from build123d import *

# Parameters (mm, degrees)
SKETCH_W       = 12
SKETCH_H       = 17.5
PAD_DEPTH      = 1.5
PAD_DEPTH_BACK = 10
SKETCH001_R    = 0.75
PAD001_DEPTH   = 10
PAD002_DEPTH   = 5
FILLET_R       = 1
FILLET001_R    = 1
FILLET002_R    = 1
SKETCH003_W    = 5.5
SKETCH003_H    = 7
PAD003_DEPTH   = 1.8
SKETCH004_R    = 2
PAD004_DEPTH   = 0.5
SKETCH005_R    = 2
PAD005_DEPTH   = 7
PAD005_TAPER   = -60


with BuildPart() as part:
    # Sketch → Pad (new body, two sides)
    with BuildSketch(Plane.XY) as pad_sk:
        Rectangle(SKETCH_W, SKETCH_H)
    extrude(amount=PAD_DEPTH)
    extrude(pad_sk.sketch, amount=-PAD_DEPTH_BACK)

    # Sketch001 → Pad001 (join)
    with BuildSketch(Plane.XY):
        with Locations((-3.25, 6)):
            Circle(SKETCH001_R)
        with Locations((-3.25, -6)):
            Circle(SKETCH001_R)
    extrude(amount=PAD001_DEPTH)

    # Sketch002 → Pad002 (join, symmetric)
    with BuildSketch(Plane.XZ):
        with BuildLine():
            ThreePointArc((16, -10), (13.071068, -2.928932), (6, 0))
            Line((6, -10), (6, 0))
            Line((16, -10), (6, -10))
        make_face()
    extrude(amount=PAD002_DEPTH, both=True)

    # Fillet
    fillet_edges = [part.edges().sort_by_distance(p)[0] for p in [
        (6, -8.75, -4.25),
        (-6, -8.75, -4.25),
        (6, 8.75, -4.25),
        (-6, 8.75, -4.25),
    ]]
    fillet(fillet_edges, radius=FILLET_R)

    # Fillet001
    fillet001_edges = [part.edges().sort_by_distance(p)[0] for p in [
        (13.071068, -5, -2.928932),
        (13.071068, 5, -2.928932),
    ]]
    fillet(fillet001_edges, radius=FILLET001_R)

    # Fillet002
    fillet002_edges = [part.edges().sort_by_distance(p)[0] for p in [
        (6, -5, -5.5),
    ]]
    fillet(fillet002_edges, radius=FILLET002_R)

    # Sketch003 (on Face6 of Fillet002) → Pad003 (join)
    with BuildSketch(Plane.XY.offset(1.5)):
        with Locations((-3.25, 0)):
            Rectangle(SKETCH003_W, SKETCH003_H)
    extrude(amount=PAD003_DEPTH)

    # Sketch004 (on Face28 of Pad003) → Pad004 (join)
    with BuildSketch(Plane.XY.offset(3.3)):
        with Locations((-3.25, -0.25)):
            Circle(SKETCH004_R)
    extrude(amount=PAD004_DEPTH)

    # Sketch005 (on Face32 of Pad004) → Pad005 (join)
    with BuildSketch(Plane.XY.offset(3.8)):
        with Locations((-3.25, -0.25)):
            Circle(SKETCH005_R)
    extrude(amount=PAD005_DEPTH, taper=PAD005_TAPER)

    # Sketch006 (on DatumPlane) → Groove (revolve, cut)
    with BuildSketch(Plane(origin=(-3.25, -0.25, 3.8), x_dir=(1, 0, 0), z_dir=(0, -1, 0))):
        Polygon((2, 0), (2, -18), (30, -18), (30, 7), (14.124356, 7), align=None)
    revolve(axis=Axis((-3.25, -0.25, 3.8), (0, 0, 1)), mode=Mode.SUBTRACT)


solid = part.part
Can you work these out from the model? Positions are in its coordinate system, mm. A direction names the side the tool comes from. Coordinates: 2 decimals unless noted, no trailing zeros. Write each loop counter-clockwise with the first axis right and the second up, starting at its lowest first coordinate (ties: lowest second). Pieces come first, ordered by that corner, then holes.
Q1. For P1, Ø1, axis at x = -4.5, y = -7.5, coming from the -Z side; P2, Ø4, axis at y = -0.5, z = 6, coming from the -X side; P3, Ø3, axis at x = -14, z = 7, coming from the +Y side; P4, Ø4, axis at x = 5.5, y = 0, coming from the -Z side, each with a flat end and sliding along its axis, tell me the tip position at first contact or that it passes through.
Results found:
P1: stops at z = 6.6
P2: stops at x = -12.52
P3: passes through
P4: stops at z = 6.54
Q2. Which directions (+Z, -Z, +X, -X, +Y, -Y) give clear straight access to the entire face, cutting with the end or side of a thin tool? Please do faces 1 (the face through (-3, 0, 10.8)), 2 (the face through (-3.7, -2.2, -3.2)).
Results found:
face 1: +Z, +X, -X, +Y, -Y
face 2: -Z
Q3. Please list where these lines run through material, in increasing order: L1, parallel to Z at x = 0.5, y = -6.5; L2, parallel to Z at x = 8.5, y = -4.25; L3, parallel to X at y = -1, z = 0.
Results found:
L1: z = 6.85 to 10.8
L2: z = 9.81 to 10.8
L3: x = -5.1 to -1.4
Q4. Imagine slicing it at A-A, the plane z = 2. List the corners of the cut face in (x, y) for me, plus the area to 3 significant figures.
Results found:
outline: circle Ø4 at (-3.25, -0.25)
area: 12.6 mm2
Q5. Imagine slicing it at B-B, the plane z = 4.5. List the corners of the cut face in (x, y) for me.
Results found:
outline: circle Ø6.42 at (-3.25, -0.25)
